Work out the finished part from the listing and answer in its coordinate system (mm). A direction names the side the tool comes from. Coordinates: 2 decimals unless noted, no trailing zeros. Write each loop counter-clockwise with the first axis right and the second up, starting at its lowest first coordinate (ties: lowest second). Pieces come first, ordered by that corner, then holes. Notation, with made-up numbers: (36.5, 17) - (82.5, 17) arc R31 ccw to (82.5, 46) - close; hole circle Ø7 at (6, -17.75). An arc over 180 degrees is marked (long way). Use a Markdown table: item, result. Add a question column.
(1) The part is cut by section D-D, the plane z = 0. Give the vertices of the cut face in (x, y).
(2) Given pin 1 Ø4.5 at (x, z) = (-70, -45) entering from -Y; pin 2 Ø3.5 at (x, z) = (20, -40) entering from +Y; pin 3 Ø0.8 at (x, y) = (-79, 19) entering from -Z; pin 4 Ø2.5 at (x, z) = (0, -40) entering from +Y, each flat-ended and moving along its own axis, determine where each tip first touches the part or whether it passes through.
(3) A tool of negligible diameter and unlimited length cuts with its end or side. For faces 4 (the face through (3.703, 5.141, 47.732)), 5 (the face through (-73, 22, 41)), 6 (the face through (-1, 0, -1)), 7 (the face through (-71.364, 2.535, -46.25)), from which of +Z, -Z, +X, -X, +Y, -Y can it reach the whole face along a straight path? Write none if from no direction.
(4) For a pull along X with two mould halves and no side action, classify faces 1 (the face through (-1, 22, 46.5)), 2 (the face through (-78.732, 14.797, 26.359)), 3 (the face through (-80, 20, 1)) as released by +X, released by -X, zero draft, split by the parting line, or undercut.
(5) The part is cut by section C-C, the plane y = 36.5. Give the vertices of the cut face in (x, z), then the cut area to 3 significant figures.
(6) Find the intervals of material crossed by line 1 (X direction, y = 3, z = 45); line 2 (Z direction, x = 20, y = 1); line 3 (Z direction, x = -70, y = 3), in increasing order. Write a range as from..to.
(7) The part is cut by section A-A, the plane x = 16. Give the vertices of the cut face in (y, z), then the cut area to 3 significant figures.
(8) The part is cut by section B-B, the plane z = -20.5. Give the vertices of the cut face in (x, y), then the cut area to 4 significant figures.
from build123d import *

# Parameters (mm, degrees)
SKETCH1_W                 = 160
SKETCH1_H                 = 98
BOSS_EXTRUDE1_DEPTH       = 40
SHELL1_T                  = -2.5
SHELL1_THICKNESS_2_FACE_W = 93
SHELL1_THICKNESS_2_FACE_H = 155
SHELL1_THICKNESS_2_DEPTH  = 1.5
CHAMFER1_SIZE             = 2
CHAMFER2_SIZE             = 10
HOLE2_START               = 28
HOLE2_OUTLINE_R           = 1.35
HOLE2_DEPTH               = 12
HOLE3_D                   = 2.7
MIRROR2_COPY_1_D          = 2.7
CUT_EXTRUDE2_REACH        = 174.049
SKETCH15_W                = 19.4
SKETCH15_H                = 13
CUT_EXTRUDE3_REACH        = 174.049
SKETCH16_W                = 20
SKETCH16_H                = 12
FILLET4_R                 = 4
SKETCH17_R                = 4
CUT_EXTRUDE4_DEPTH        = 133.680066325
SKETCH20_W                = 30
SKETCH20_H                = 12
CUT_EXTRUDE5_DEPTH        = 157.939807062
FILLET6_R                 = 4


# Read off the part's stored shape, not the designer's step: Hole1, Hole2
with BuildPart() as part:
    # Sketch1 → Boss-Extrude1 (new body)
    with BuildSketch(Plane(origin=(0, 0, 0), x_dir=(1, 0, 0), z_dir=(0, 1, 0))):
        Rectangle(SKETCH1_W, SKETCH1_H)
    extrude(amount=BOSS_EXTRUDE1_DEPTH)

    # Shell1
    shell1_openings = [part.faces().sort_by_distance(p)[0] for p in [
        (0, 40, 0),
    ]]
    offset(amount=SHELL1_T, openings=shell1_openings, kind=Kind.INTERSECTION)

    # Shell1 thickness 2 face (on inner face of the shell) → Shell1 thickness 2 (add)
    with BuildSketch(Plane(origin=(0, 2.5, 0), x_dir=(0, 0, -1), z_dir=(0, -1, 0))):
        Rectangle(SHELL1_THICKNESS_2_FACE_W, SHELL1_THICKNESS_2_FACE_H)
    extrude(amount=-SHELL1_THICKNESS_2_DEPTH)

    # Chamfer1
    chamfer1_edges = [part.edges().sort_by_distance(p)[0] for p in [
        (80, 20, 49),
        (-80, 20, 49),
        (-80, 20, -49),
        (80, 20, -49),
    ]]
    chamfer(chamfer1_edges, length=CHAMFER1_SIZE)

    # Chamfer2
    chamfer2_edges = [part.edges().sort_by_distance(p)[0] for p in [
        (77.5, 22, 46.5),
        (77.5, 22, -46.5),
        (-77.5, 22, -46.5),
        (-77.5, 22, 46.5),
    ]]
    chamfer(chamfer2_edges, length=CHAMFER2_SIZE)

    # Hole1 outline → Hole1 (revolve, cut)
    with BuildSketch(Plane(origin=(-70, 0, 45), x_dir=(1, 0, 0), z_dir=(0, 0, 1))):
        Polygon((1.85, 0), (1.85, 5), (0, 6.85), (0, 0), align=None)
    revolve(axis=Axis((-70, 0, 45), (0, 1, 0)), mode=Mode.SUBTRACT)

    # Hole1 2 outline → Hole1 2 (revolve, cut)
    with BuildSketch(Plane(origin=(70, 0, -45), x_dir=(1, 0, 0), z_dir=(0, 0, 1))):
        Polygon((1.85, 0), (1.85, 5), (0, 6.85), (0, 0), align=None)
    revolve(axis=Axis((70, 0, -45), (0, 1, 0)), mode=Mode.SUBTRACT)

    # Hole1 3 outline → Hole1 3 (revolve, cut)
    with BuildSketch(Plane(origin=(70, 0, 45), x_dir=(1, 0, 0), z_dir=(0, 0, 1))):
        Polygon((1.85, 0), (1.85, 5), (0, 6.85), (0, 0), align=None)
    revolve(axis=Axis((70, 0, 45), (0, 1, 0)), mode=Mode.SUBTRACT)

    # Hole1 4 outline → Hole1 4 (revolve, cut)
    with BuildSketch(Plane(origin=(-70, 0, -45), x_dir=(1, 0, 0), z_dir=(0, 0, 1))):
        Polygon((1.85, 0), (1.85, 5), (0, 6.85), (0, 0), align=None)
    revolve(axis=Axis((-70, 0, -45), (0, 1, 0)), mode=Mode.SUBTRACT)

    # Hole2 outline → Hole2 (cut)
    with BuildSketch(Plane(origin=(0, 0, 0), x_dir=(1, 0, 0), z_dir=(0, 1, 0)).offset(HOLE2_START)):
        with Locations((76, -45)):
            Circle(HOLE2_OUTLINE_R)
        with Locations((-76, 45)):
            Circle(HOLE2_OUTLINE_R)
        with Locations((-76, -45)):
            Circle(HOLE2_OUTLINE_R)
        with Locations((76, 45)):
            Circle(HOLE2_OUTLINE_R)
    extrude(amount=HOLE2_DEPTH, mode=Mode.SUBTRACT)

    # Hole3 (through all)
    with Locations(Plane(origin=(0, 4, 0), x_dir=(1, 0, 0), z_dir=(0, 1, 0))):
        with Locations((60, -40), (0, -40), (20, -40), (40, -40)):
            hole3 = Hole(HOLE3_D / 2)

    # Mirror1: Hole3 across plane
    add(hole3.mirror(Plane(origin=(0, 0, 0), x_dir=(0, 0, 1), z_dir=(1, 0, 0))), mode=Mode.SUBTRACT)

    # Mirror2: Hole3 across plane
    add(hole3.mirror(Plane.XY), mode=Mode.SUBTRACT)

    # Mirror2 copy 1 (through all)
    with Locations(Plane(origin=(0, 4, 0), x_dir=(-1, 0, 0), z_dir=(0, 1, 0))):
        with Locations((60, -40), (0, -40), (20, -40), (40, -40)):
            Hole(MIRROR2_COPY_1_D / 2)

    # Sketch15 → Cut-Extrude2 (cut, up to next)
    with BuildSketch(Plane.ZY.offset(80), mode=Mode.PRIVATE) as cut_extrude2_sk1:
        with Locations((-25, 20)):
            Rectangle(SKETCH15_W, SKETCH15_H)
    cut_extrude2_tool1 = extrude(cut_extrude2_sk1.sketch, amount=-CUT_EXTRUDE2_REACH, mode=Mode.PRIVATE) & part.part
    add(cut_extrude2_tool1.solids().sort_by_distance((-80, 20, -25))[0], mode=Mode.SUBTRACT)

    # Sketch16 → Cut-Extrude3 (cut, up to next)
    with BuildSketch(Plane.ZY.offset(80), mode=Mode.PRIVATE) as cut_extrude3_sk1:
        with Locations((17.5, 10)):
            Rectangle(SKETCH16_W, SKETCH16_H)
    cut_extrude3_tool1 = extrude(cut_extrude3_sk1.sketch, amount=-CUT_EXTRUDE3_REACH, mode=Mode.PRIVATE) & part.part
    add(cut_extrude3_tool1.solids().sort_by_distance((-80, 10, 17.5))[0], mode=Mode.SUBTRACT)

    # Fillet4
    fillet4_edges = [part.edges().sort_by_distance(p)[0] for p in [
        (-78.75, 16, 7.5),
        (-78.75, 4, 7.5),
        (-78.75, 4, 27.5),
        (-78.75, 16, 27.5),
    ]]
    fillet(fillet4_edges, radius=FILLET4_R)

    # Sketch17 → Cut-Extrude4 (cut, through all)
    with BuildSketch(Plane.XY.offset(49)):
        with Locations((40, 28)):
            Circle(SKETCH17_R)
    extrude(amount=-CUT_EXTRUDE4_DEPTH, mode=Mode.SUBTRACT)

    # Sketch20 → Cut-Extrude5 (cut, through all)
    with BuildSketch(Plane(origin=(35.971952471, 0.293460479, 49), x_dir=(1, 0, 0), z_dir=(0, 0, 1))):
        with Locations((-18.471952471, 9.706539521)):
            Rectangle(SKETCH20_W, SKETCH20_H)
    extrude(amount=-CUT_EXTRUDE5_DEPTH, mode=Mode.SUBTRACT)

    # Fillet6
    fillet6_edges = [part.edges().sort_by_distance(p)[0] for p in [
        (2.5, 16, -47.75),
        (32.5, 16, -47.75),
        (2.5, 4, -47.75),
        (32.5, 4, -47.75),
        (32.5, 4, 47.75),
        (32.5, 16, 47.75),
        (2.5, 4, 47.75),
        (2.5, 16, 47.75),
    ]]
    fillet(fillet6_edges, radius=FILLET6_R)


solid = part.part
Model answer:
| question | item | result |
|---|---|---|
| 1 | outline | (-80, 0) - (80, 0) - (80, 40) - (77.5, 40) - (77.5, 4) - (-77.5, 4) - (-77.5, 40) - (-80, 40) - close |
| 2 | pin 1 | y = 0 |
| 2 | pin 2 | y = 4 |
| 2 | pin 3 | z = -48.4 |
| 2 | pin 4 | through |
| 3 | face 4 | +Z, -Z |
| 3 | face 5 | +Y |
| 3 | face 6 | +Z, -Z, +X, -X, -Y |
| 3 | face 7 | -Y |
| 4 | face 1 | undercut |
| 4 | face 2 | zero draft |
| 4 | face 3 | released by -X |
| 5 | outline | (-80, -47) - (-78, -49) - (78, -49) - (80, -47) - (80, 47) - (78, 49) - (-78, 49) - (-80, 47) - close; hole (-77.5, -36.5) - (-67.5, -46.5) - (67.5, -46.5) - (77.5, -36.5) - (77.5, 36.5) - (67.5, 46.5) - (-67.5, 46.5) - (-77.5, 36.5) - close; hole circle Ø2.7 at (-76, -45); hole circle Ø2.7 at (-76, 45); hole circle Ø2.7 at (76, -45); hole circle Ø2.7 at (76, 45) |
| 5 | area | 1,430 mm^2 |
| 6 | line 1 | -80..-71.85, -68.15..68.15, 71.85..80 |
| 6 | line 2 | -49..-41.35, -38.65..38.65, 41.35..49 |
| 6 | line 3 | -49..-46.85, -43.15..43.15, 46.85..49 |
| 7 | outline | (0, -49) - (4, -49) - (4, 49) - (0, 49) - close; (16, -49) - (40, -49) - (40, -46.5) - (16, -46.5) - close; (16, 46.5) - (40, 46.5) - (40, 49) - (16, 49) - close |
| 7 | area | 512 mm^2 |
| 8 | outline | (-80, 0) - (80, 0) - (80, 40) - (77.5, 40) - (77.5, 4) - (-77.5, 4) - (-77.5, 13.5) - (-80, 13.5) - close; (-80, 26.5) - (-77.5, 26.5) - (-77.5, 40) - (-80, 40) - close |
| 8 | area | 787.5 mm^2 |
